Autodesk Inventor part; units mm, degrees
ref_plane "YZ Plane" through (0, 0, 0) normal (1, 0, 0) x (0, 1, 0)
ref_plane "XZ Plane" through (0, 0, 0) normal (0, 1, 0) x (-1, 0, 0)
ref_plane "XY Plane" through (0, 0, 0) normal (0, 0, 1) x (1, 0, 0)
sketch "スケッチ1" plane through (0, 0, 0) normal (0, 1, 0) x (-1, 0, 0)
  line L0 (0, 0) -> (95, 0)
  line L1 (95, 0) -> (95, -72)
  line L2 (95, -72) -> (0, -72)
  line L3 (0, -72) -> (0, 0)
  dimension "d0" = 95
  dimension "d1" = 72
extrude "押し出し1" add sketch "スケッチ1" along normal blind 1
hole "穴1" at (-92, 1, -3) direction (0, -1, 0) diameter 3 end through all
hole "穴2" at (-92, 1, -69) direction (0, -1, 0) diameter 3 end through all
hole "穴3" at (-3, 1, -3) direction (0, -1, 0) diameter 3 end through all
hole "穴4" at (-3, 1, -69) direction (0, -1, 0) diameter 3 end through all
properties part number "基板"
Design review of the part built by this model. Coordinates are the model's own, in mm. Give positions to 0.01 mm unless a question says otherwise; leave off trailing zeros. Order: outer loops, then holes, each group sorted by start corner. A loop starts at its lowest first (then second) coordinate and runs counter-clockwise, first axis right, second up. Notation, with made-up numbers: (58, 77.25) - (104, 77.25) arc R13 ccw to (104, 92.25) - close; hole circle Ø9 at (0, 65.25). An arc over 180 degrees is marked (long way). Use a Markdown table: item, result. Add a question column.
(1) Add section B-B on x = -3. Give the boundary of the cut face in (y, z).
(2) Wall thickness on probe 1 along Z at (x, y) = (-92, 0.65); probe 2 along X at (y, z) = (0.65, -3): over which ranges is each line inside the solid? List them lowest first. Write a range as [from, to].
(3) Add section A-A on z = -3. Give the boundary of the cut face in (x, y), then the cut area to 3 significant figures.
(4) Mouldability with a two-part tool opening along X and no side actions: class faces 1 (the face through (-47, 1, -35)), 2 (the face through (-3.45, 0.49, -67.57)) as +X half, -X half, draft (parallel to the pull), parting line (faces both ways), or undercut.
Report:
| question | item | result |
|---|---|---|
| 1 | outline | (0, -72) - (1, -72) - (1, -70.5) - (0, -70.5) - close; (0, -67.5) - (1, -67.5) - (1, -4.5) - (0, -4.5) - close; (0, -1.5) - (1, -1.5) - (1, 0) - (0, 0) - close |
| 2 | probe 1 | z = [-72, -70.5], [-67.5, -4.5], [-1.5, 0] |
| 2 | probe 2 | x = [-95, -93.5], [-90.5, -4.5], [-1.5, 0] |
| 3 | outline | (-95, 0) - (-93.5, 0) - (-93.5, 1) - (-95, 1) - close; (-90.5, 0) - (-4.5, 0) - (-4.5, 1) - (-90.5, 1) - close; (-1.5, 0) - (0, 0) - (0, 1) - (-1.5, 1) - close |
| 3 | area | 89.0 mm² |
| 4 | face 1 | draft |
| 4 | face 2 | undercut |
